Read the model definition and answer for the solid it produces. Units are mm, in the model's axes. Give positions to 0.01 mm unless a question says otherwise; leave off trailing zeros. Order: outer loops, then holes, each group sorted by start corner. A loop starts at its lowest first (then second) coordinate and runs counter-clockwise, first axis right, second up.
Item 1: The mould has two halves that part along Y. Classify faces 1 (the face through (0.067, 19.191, -34.903)), 2 (the face through (-4.762, 0, 1)), 3 (the face through (0, -25.4, 1)): +Y half, -Y half, draft (parallel to the pull), parting line (faces both ways), or undercut.
Item 2: A cutting plane is placed at B-B (z = -37). Write down the section's boundary in (x, y) (1 decimal).
Item 3: A cutting plane is placed at D-D (z = 38.1). Write down the section's boundary in (x, y).
Item 4: A cutting plane is placed at C-C (x = 3.5). Write down the section's boundary in (y, z).
Item 5: Given pin 1 Ø6 at (y, z) = (-17.88, 37) entering from +X, flat-ended and moving along its own axis, determine where the tip first touches the part or whether it passes through.
Item 6: Find the intervals of material crossed by line 1 along Y through (x, z) = (-2, -38.1); line 2 along Y through (x, z) = (0.25, 38.1); line 3 along Y through (x, z) = (-2.5, 41), in increasing order.
Item 7: A cutting plane is placed at A-A (y = 19.05). Write down the section's boundary in (x, z), plus the area to 3 significant figures.
from build123d import *

# Parameters (mm, degrees)
SKETCH1_W           = 88.9
SKETCH1_H           = 50.8
BOSS_EXTRUDE1_DEPTH = 4.7625
SKETCH2_R           = 3.2
CUT_EXTRUDE1_DEPTH  = 10.525
FILLET3_R           = 2.54
FILLET4_R           = 2.54
SKETCH4_R           = 3.2
CUT_EXTRUDE5_DEPTH  = 10.525


with BuildPart() as part:
    # Sketch1 → Boss-Extrude1 (new body, symmetric)
    with BuildSketch(Plane(origin=(0, 0, 0), x_dir=(0, 0, -1), z_dir=(1, 0, 0))):
        Rectangle(SKETCH1_W, SKETCH1_H)
    extrude(amount=BOSS_EXTRUDE1_DEPTH, both=True)

    # Sketch2 → Cut-Extrude1 (cut, through all)
    with BuildSketch(Plane(origin=(4.7625, 0, 0), x_dir=(0, 0, -1), z_dir=(1, 0, 0))):
        with Locations((-38.1, 19.05)):
            Circle(SKETCH2_R)
        with Locations((38.1, 19.05)):
            Circle(SKETCH2_R)
        with Locations((-38.1, -4)):
            Circle(SKETCH2_R)
        with Locations((38.1, -4)):
            Circle(SKETCH2_R)
    extrude(amount=-CUT_EXTRUDE1_DEPTH, mode=Mode.SUBTRACT)

    # Fillet3
    fillet3_edges = [part.edges().sort_by_distance(p)[0] for p in [
        (0, 25.4, 44.45),
    ]]
    fillet(fillet3_edges, radius=FILLET3_R)

    # Fillet4
    fillet4_edges = [part.edges().sort_by_distance(p)[0] for p in [
        (0, 25.4, -44.45),
    ]]
    fillet(fillet4_edges, radius=FILLET4_R)

    # Sketch4 → Cut-Extrude5 (cut, through all)
    with BuildSketch(Plane(origin=(4.7625, 0, 0), x_dir=(0, 0, -1), z_dir=(1, 0, 0))):
        with Locations((-37.002111381, -17.879327913)):
            Circle(SKETCH4_R)
        with Locations((38.440338437, -17.879327913)):
            Circle(SKETCH4_R)
    extrude(amount=-CUT_EXTRUDE5_DEPTH, mode=Mode.SUBTRACT)


solid = part.part
Response values:
1. face 1: undercut
1. face 2: draft
1. face 3: -Y half
2. outline: (-4.8, -25.4) - (4.8, -25.4) - (4.8, -20.7) - (-4.8, -20.7) - close; (-4.8, -15) - (4.8, -15) - (4.8, -7) - (-4.8, -7) - close; (-4.8, -1) - (4.8, -1) - (4.8, 16) - (-4.8, 16) - close; (-4.8, 22.1) - (4.8, 22.1) - (4.8, 25.4) - (-4.8, 25.4) - close
3. outline: (-4.76, -25.4) - (4.76, -25.4) - (4.76, -20.89) - (-4.76, -20.89) - close; (-4.76, -14.87) - (4.76, -14.87) - (4.76, -7.2) - (-4.76, -7.2) - close; (-4.76, -0.8) - (4.76, -0.8) - (4.76, 15.85) - (-4.76, 15.85) - close; (-4.76, 22.25) - (4.76, 22.25) - (4.76, 25.4) - (-4.76, 25.4) - close
4. outline: (-25.4, -44.45) - (22.86, -44.45) arc R2.54 ccw to (25.4, -41.91) - (25.4, 41.91) arc R2.54 ccw to (22.86, 44.45) - (-25.4, 44.45) - close; hole circle Ø6.4 at (-17.88, -38.44); hole circle Ø6.4 at (-17.88, 37); hole circle Ø6.4 at (-4, -38.1); hole circle Ø6.4 at (-4, 38.1); hole circle Ø6.4 at (19.05, -38.1); hole circle Ø6.4 at (19.05, 38.1)
5. pin 1: passes through
6. line 1: y = -25.4 to -21.06, -14.7 to -7.2, -0.8 to 15.85, 22.25 to 25.4
6. line 2: y = -25.4 to -20.89, -14.87 to -7.2, -0.8 to 15.85, 22.25 to 25.4
6. line 3: y = -25.4 to -5.35, -2.65 to 17.7, 20.4 to 25.4
7. outline: (-4.76, -44.45) - (4.76, -44.45) - (4.76, -41.3) - (-4.76, -41.3) - close; (-4.76, -34.9) - (4.76, -34.9) - (4.76, 34.9) - (-4.76, 34.9) - close; (-4.76, 41.3) - (4.76, 41.3) - (4.76, 44.45) - (-4.76, 44.45) - close
7. area: 725 mm2
